from build123d import *

# Parameters (mm, degrees)
SKIZZE1_R                       = 100
SKIZZE1_R_2                     = 60
BASIS_LINEAR_AUSTRAGEN_DEPTH    = 40
SCHNITT_LINEAR_AUSTRAGEN1_DEPTH = 20
SKIZZE4_R                       = 0.5
SCHNITT_LINEAR_AUSTRAGEN3_DEPTH = 41
M6X1_0_GEWINDEKERNLOCH1_D       = 5


with BuildPart() as part:
    # Skizze1 → Basis-Linear austragen (new body)
    with BuildSketch(Plane.XY):
        Circle(SKIZZE1_R)
        with Locations((0, 7.5)):
            Circle(SKIZZE1_R_2, mode=Mode.SUBTRACT)
    extrude(amount=BASIS_LINEAR_AUSTRAGEN_DEPTH)

    # Skizze2 → Schnitt-Linear austragen1 (cut)
    with BuildSketch(Plane.XY.offset(40)):
        with BuildLine():
            Line((17.272249399, -45.127588459), (52.627588459, -9.772249399))
            Line((52.627588459, -9.772249399), (74.246212025, -31.390872965))
            ThreePointArc((74.246212025, -31.390872965), (77.175144213, -38.461940777), (74.246212025, -45.533008589))
            Line((74.246212025, -45.533008589), (53.033008589, -66.746212025))
            ThreePointArc((53.033008589, -66.746212025), (45.961940777, -69.675144213), (38.890872965, -66.746212025))
            Line((38.890872965, -66.746212025), (17.272249399, -45.127588459))
        make_face()
    extrude(amount=-SCHNITT_LINEAR_AUSTRAGEN1_DEPTH, mode=Mode.SUBTRACT)

    # Skizze4 → Schnitt-Linear austragen3 (cut, through all)
    with BuildSketch(Plane.XY.offset(40)):
        with Locations((-1, -64.992307237)):
            Circle(SKIZZE4_R)
    extrude(amount=-SCHNITT_LINEAR_AUSTRAGEN3_DEPTH, mode=Mode.SUBTRACT)

    # M6x1.0 Gewindekernloch1 (through all)
    with Locations(Plane.XY.offset(20)):
        with Locations((45.961940777, -59.675144213), (67.175144213, -38.461940777)):
            Hole(M6X1_0_GEWINDEKERNLOCH1_D / 2)


solid = part.part
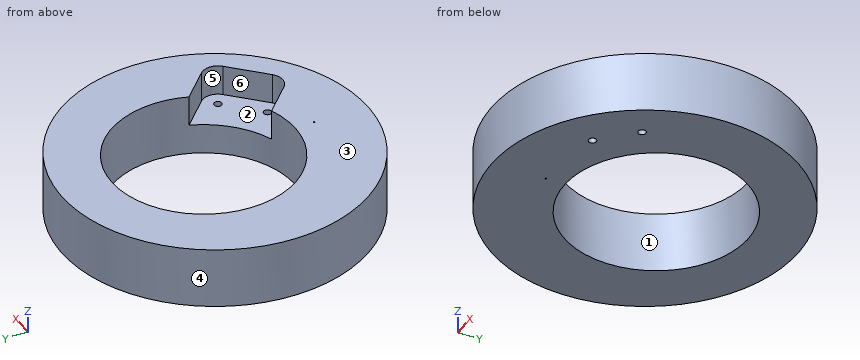
CAD build for the part. Positions are in the model's coordinates, mm. Face numbers are marked on the shaded views. A direction names the side the tool comes from. Give positions to 0.01 mm unless a question says otherwise; leave off trailing zeros. Order: outer loops, then holes, each group sorted by start corner. A loop starts at its lowest first (then second) coordinate and runs counter-clockwise, first axis right, second up. Notation, with made-up numbers: (-3, 83) - (18, 83) arc R16 ccw to (18, 98) - close; hole circle Ø9 at (42, 13). An arc over 180 degrees is marked (long way). Answer in a Markdown table with one row per item.
1. Saw through at A-A, the plane x = -6.5. Give the cut face in (y, z).
Data:
| item | result |
|---|---|
| outline | (-99.79, 0) - (-52.15, 0) - (-52.15, 40) - (-99.79, 40) - close; (67.15, 0) - (99.79, 0) - (99.79, 40) - (67.15, 40) - close |
2. Saw through at B-B, the plane y = 7.5. Give the cut face in (x, z).
Data:
| item | result |
|---|---|
| outline | (-99.72, 0) - (-60, 0) - (-60, 40) - (-99.72, 40) - close; (60, 0) - (99.72, 0) - (99.72, 40) - (60, 40) - close |
3. Pull direction Y, two halves, no side cores. Call the marked faces 3, 4, 5 and 6: pulls with the +Y half, pulls with the -Y half, needs draft (parallel to the pull), parting line crosses it, or undercut.
Data:
| item | result |
|---|---|
| face 3 | needs draft |
| face 4 | parting line crosses it |
| face 5 | undercut |
| face 6 | undercut |
4. Saw through at C-C, the plane z = 37.5. Give the cut face in (x, y).
Data:
| item | result |
|---|---|
| outline | circle Ø200 at (0, 0); hole circle Ø1 at (-1, -64.99); hole (20.89, -48.75) - (38.89, -66.75) arc R10 ccw to (53.03, -66.75) - (74.25, -45.53) arc R10 ccw to (74.25, -31.39) - (56.25, -13.39) arc R60 ccw (long way) to start |
5. Saw through at D-D, the plane x = 67. Give the cut face in (y, z).
Data:
| item | result |
|---|---|
| outline | (-74.24, 0) - (-40.96, 0) - (-40.96, 20) - (-52.78, 20) - (-52.78, 40) - (-74.24, 40) - close; (-35.97, 0) - (74.24, 0) - (74.24, 40) - (-24.14, 40) - (-24.14, 20) - (-35.97, 20) - close |
6. Probe probe 1 along Y at (x, z) = (-1, 26.5) (3 decimals); probe 2 along Y at (x, z) = (8, 37.5); probe 3 along X at (y, z) = (-31.5, 28). List the from-to ranges inside material, lowest first. Write a range as [from, to].
Data:
| item | result |
|---|---|
| probe 1 | y = [-99.995, -65.492], [-64.492, -52.492], [67.492, 99.995] |
| probe 2 | y = [-99.68, -51.96], [66.96, 99.68] |
| probe 3 | x = [-94.91, -45.6], [74.35, 94.91] |
7. Tool access for the marked faces 1 and 2: list every direction of +Z, -Z, +X, -X, +Y, -Y with a clear straight run to the whole face (end or side of a thin tool).
Data:
| item | result |
|---|---|
| face 1 | +Z, -Z |
| face 2 | +Z |
8. Flat gauge pins, fed straight in: pin 1 (4.5 mm diameter, centred on x = 67.18, y = -38.46, fed in from -Z); pin 2 (1 mm diameter, centred on x = 66, z = 5.5, fed in from -Y); pin 3 (3 mm diameter, centred on y = 23.5, z = 4, fed in from +X); pin 4 (5 mm diameter, centred on x = 55.5, z = 9, fed in from +Y). Where does each tip first touch, or does it go through?
Data:
| item | result |
|---|---|
| pin 1 | passes through |
| pin 2 | stops at y = -75.56 |
| pin 3 | stops at x = 97.55 |
| pin 4 | stops at y = 84.8 |
